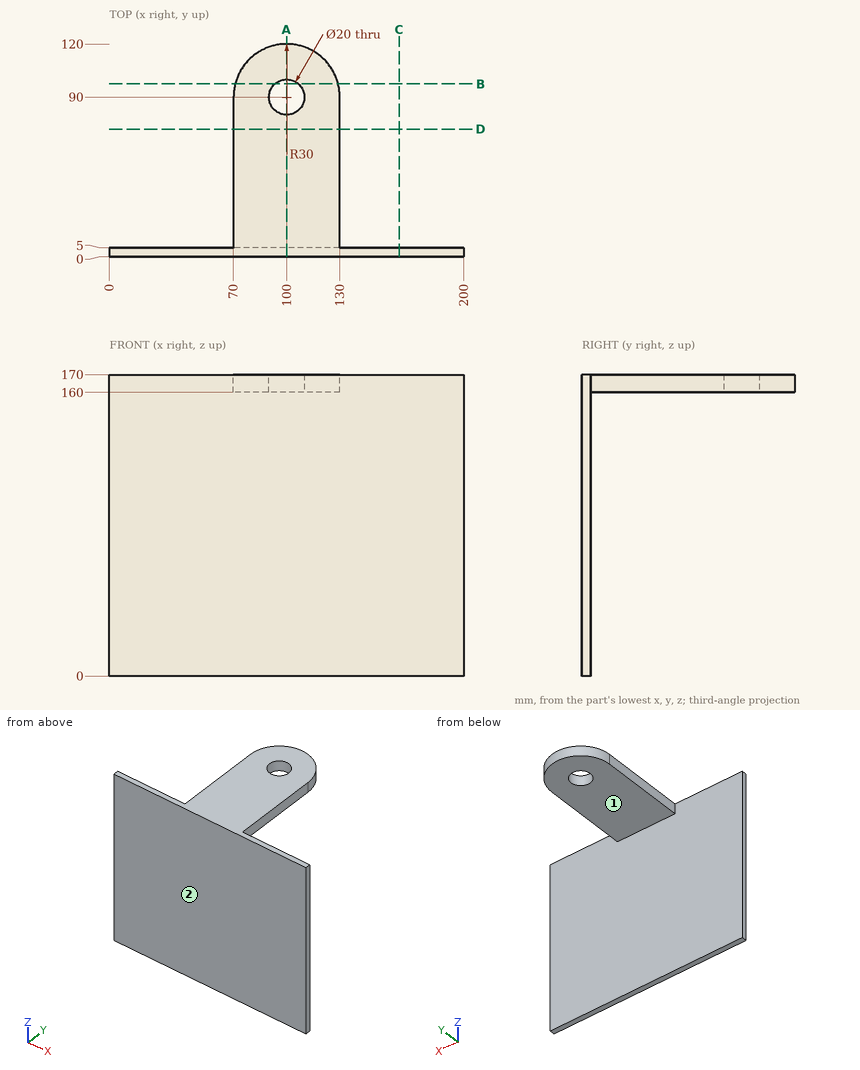
Input: dimensioned drawing with shaded views. Units: mm. Origin: part minimum x, y, z. A direction names the side the tool comes from. Give positions to 0.01 mm unless a question says otherwise; leave off trailing zeros. Loops run counter-clockwise (first coordinate to the right, second up) from the corner with the lowest first, then second, coordinate; pieces in that order, holes last. Notation, with made-up numbers: (-30, 33.5) -> (-26, 33.5) arc R11 cw to (-26, 53.5) -> close; hole circle Ø4 at (65, 71). An arc over 180 degrees is marked (long way). Use a Markdown table: item, result.
Q1. Section query A-A, the plane x = 100. Return the cut outline in (y, z), plus the area to 3 significant figures.
Entries:
| item | result |
|---|---|
| outline | (0, 0) -> (5, 0) -> (5, 160) -> (80, 160) -> (80, 170) -> (0, 170) -> close; (100, 160) -> (120, 160) -> (120, 170) -> (100, 170) -> close |
| area | 1,800 mm² |
Q2. Section query D-D, the plane y = 72. Return the cut outline in (x, z), plus the area to 3 significant figures.
Entries:
| item | result |
|---|---|
| outline | (70, 160) -> (130, 160) -> (130, 170) -> (70, 170) -> close |
| area | 600 mm² |
Q3. First-contact query: P1, Ø4, axis at x = 71.5, z = 144, coming from the +Y side; P2, Ø11, axis at y = 43.5, z = 163, coming from the +X side; P3, Ø3, axis at y = 54.5, z = 163.5, coming from the -X side. Flat tips, straight axial feed; report the tip coordinate or a pass-through.
Entries:
| item | result |
|---|---|
| P1 | stops at y = 5 |
| P2 | stops at x = 130 |
| P3 | stops at x = 70 |
Q4. Access query for the marked faces 1 and 2. Directions: +Z, -Z, +X, -X, +Y, -Y. A direction counts if a zero-diameter tool reaches every point of the face in a straight line with its end or side. Return the directions, or none.
Entries:
| item | result |
|---|---|
| face 1 | -Z, +X, -X, +Y |
| face 2 | +Z, -Z, +X, -X, -Y |
Q5. Ray query, probe 1 along Y at (x, z) = (100, 166.5); probe 2 along Z at (x, y) = (120.5, 79.5); probe 3 along Y at (x, z) = (25, 145.5). Return the intervals inside material, ascending. Write a range as from..to.
Entries:
| item | result |
|---|---|
| probe 1 | y = 0..80, 100..120 |
| probe 2 | z = 160..170 |
| probe 3 | y = 0..5 |
Q6. Section query C-C, the plane x = 163.5. Return the cut outline in (y, z), plus the area to 3 significant figures.
Entries:
| item | result |
|---|---|
| outline | (0, 0) -> (5, 0) -> (5, 170) -> (0, 170) -> close |
| area | 850 mm² |
Q7. Section query B-B, the plane y = 97.5. Return the cut outline in (x, z), plus the area to 3 significant figures.
Entries:
| item | result |
|---|---|
| outline | (70.95, 160) -> (93.39, 160) -> (93.39, 170) -> (70.95, 170) -> close; (106.61, 160) -> (129.05, 160) -> (129.05, 170) -> (106.61, 170) -> close |
| area | 449 mm² |
